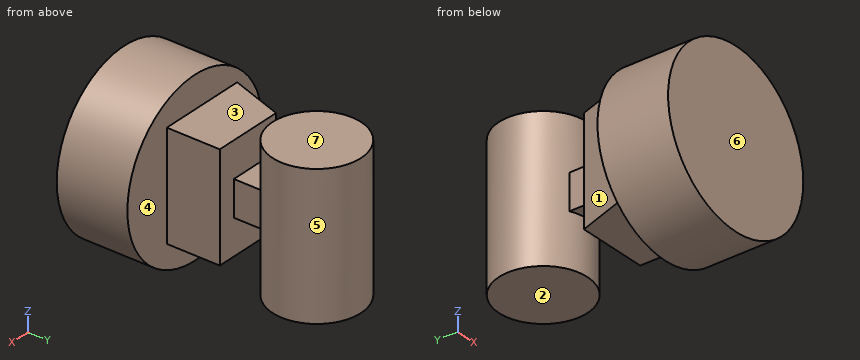
```python
from build123d import *

# Parameters (mm, degrees)
SKETCH1_R           = 24
BOSS_EXTRUDE1_DEPTH = 20
SKETCH4_R           = 12.5
BOSS_EXTRUDE3_DEPTH = 20
BOSS_EXTRUDE5_DEPTH = 15
SKETCH6_W           = 10
SKETCH6_H           = 10
BOSS_EXTRUDE6_DEPTH = 8.043561


with BuildPart() as part:
    # Sketch1 → Boss-Extrude1 (new body)
    with BuildSketch(Plane(origin=(0, 0, 0), x_dir=(1, 0, 0), z_dir=(0, 1, 0))):
        Circle(SKETCH1_R)
    extrude(amount=BOSS_EXTRUDE1_DEPTH)

    # Sketch5 → Boss-Extrude5 (add, symmetric)
    with BuildSketch(Plane.XY):
        Polygon((-15, 20), (10, 20), (10, 35), (-10, 35), align=None)
    extrude(amount=BOSS_EXTRUDE5_DEPTH, both=True)



with BuildPart() as body_2:
    # Sketch4 → Boss-Extrude3 (new body, symmetric)
    with BuildSketch(Plane.XY):
        with Locations((0, 54.5)):
            Circle(SKETCH4_R)
    extrude(amount=BOSS_EXTRUDE3_DEPTH, both=True)


with BuildPart() as part_1:
    add(part.part)

    add(body_2.part)  # Boss-Extrude6 merges body 2
    # Sketch6 → Boss-Extrude6 (add)
    with BuildSketch(Plane(origin=(0, 35, 0), x_dir=(1, 0, 0), z_dir=(0, 1, 0))):
        Rectangle(SKETCH6_W, SKETCH6_H)
    extrude(amount=BOSS_EXTRUDE6_DEPTH)


solid = part_1.part
```
The model under review builds one solid part; all positions refer to its coordinate system, in mm. Face numbers are marked on the shaded views. A direction names the side the tool comes from. Coordinates: 2 decimals unless noted, no trailing zeros. Order: outer loops, then holes, each group sorted by start corner. A loop starts at its lowest first (then second) coordinate and runs counter-clockwise, first axis right, second up. Notation, with made-up numbers: (29, 63) -> (52, 63) arc R14 ccw to (52, 87) -> close; hole circle Ø10 at (43.25, 36.25). An arc over 180 degrees is marked (long way). Answer in a Markdown table with one row per item. Add a question column.
Item 1: Machinability: for the marked faces 1, 2, 3 and 4, which of the approach directions +Z, -Z, +X, -X, +Y, -Y give a long, thin tool a straight path to every point of the face, cutting with its end or side? Answer none if there is none.
Item 2: We need section A-A on z = 0. Write out the cut boundary in (x, y).
Item 3: We need section C-C on z = -12. Write out the cut boundary in (x, y), plus the area to 3 significant figures.
Item 4: We need section B-B on x = 0. Write out the cut boundary in (y, z), plus the area to 3 significant figures.
Item 5: Mouldability with a two-part tool opening along Y and no side actions: class the marked faces 5, 6 and 7 as +Y half, -Y half, draft (parallel to the pull), parting line (faces both ways), or undercut.
Item 6: We need section D-D on y = 54.5. Write out the cut boundary in (x, z), plus the area to 3 significant figures.
Item 7: Clearance check with flat-ended pins moving along their axes: pin 1 (6 mm diameter, centred on x = -9.5, y = 37.5, fed in from +Z); pin 2 (6 mm diameter, centred on x = 17.5, y = 12.5, fed in from +Z); pin 3 (1 mm diameter, centred on y = 25.5, z = -7, fed in from -X). State where each tip first meets the part, or that it passes through.
Item 8: To check wall thickness, follow probe 1 along Y at (x, z) = (0, -18); probe 2 along Y at (x, z) = (0, 13); probe 3 along Z at (x, y) = (-9, 57). State the ranges of each line that lie inside material, in increasing order.
Final values:
| question | item | result |
|---|---|---|
| 1 | face 1 | +Z, -Z, -X |
| 1 | face 2 | -Z, +X, -X, +Y |
| 1 | face 3 | +Z, +X, -X |
| 1 | face 4 | none |
| 2 | outline | (-24, 0) -> (24, 0) -> (24, 20) -> (10, 20) -> (10, 35) -> (5, 35) -> (5, 43.04) arc R12.5 ccw (long way) to (-5, 43.04) -> (-5, 35) -> (-10, 35) -> (-15, 20) -> (-24, 20) -> close |
| 3 | outline | (-20.78, 0) -> (20.78, 0) -> (20.78, 20) -> (10, 20) -> (10, 35) -> (-10, 35) -> (-15, 20) -> (-20.78, 20) -> close; circle Ø25 at (0, 54.5) |
| 3 | area | 1,660 mm2 |
| 4 | outline | (0, -24) -> (20, -24) -> (20, -15) -> (35, -15) -> (35, -5) -> (42, -5) -> (42, -20) -> (67, -20) -> (67, 20) -> (42, 20) -> (42, 5) -> (35, 5) -> (35, 15) -> (20, 15) -> (20, 24) -> (0, 24) -> close |
| 4 | area | 2,480 mm2 |
| 5 | face 5 | undercut |
| 5 | face 6 | -Y half |
| 5 | face 7 | draft |
| 6 | outline | (-12.5, -20) -> (12.5, -20) -> (12.5, 20) -> (-12.5, 20) -> close |
| 6 | area | 1,000 mm2 |
| 7 | pin 1 | stops at z = 15 |
| 7 | pin 2 | stops at z = 19.12 |
| 7 | pin 3 | stops at x = -13.33 |
| 8 | probe 1 | y = 0 to 20, 42 to 67 |
| 8 | probe 2 | y = 0 to 35, 42 to 67 |
| 8 | probe 3 | z = -20 to 20 |
